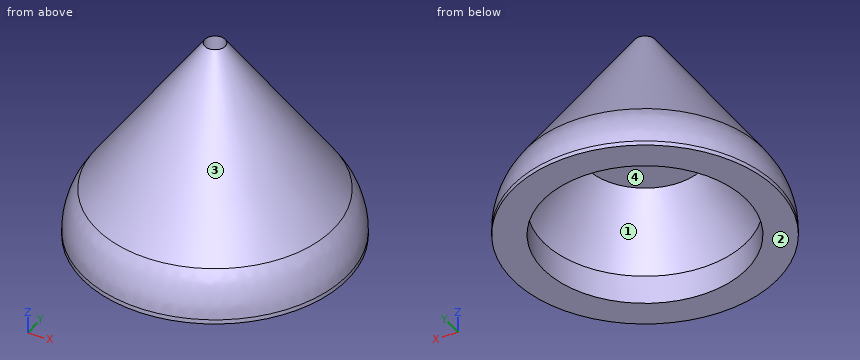
from build123d import *

# Parameters (mm, degrees)
FILLET1_R = 48.26


with BuildPart() as part:
    # Sketch2 → Revolve1 (revolve)
    with BuildSketch(Plane.YZ, mode=Mode.PRIVATE) as revolve1_sk:
        Polygon((-63.5, 0), (-63.5, 17.927965037), (-36.337085401, 56.808731059), (-6.35, 56.808731059), (-6.35, 69.508731059), (-27.464600347, 69.508731059), (-6.35, 99.731991259), (-6.35, 127), (-82.55, 17.927965037), (-82.55, 0), align=None)
    revolve(revolve1_sk.sketch.rotate(Axis((0, 0, 0), (0, 0, 1)), 270), axis=Axis((0, 0, 0), (0, 0, 1)))

    # Fillet1
    fillet1_edges = [part.edges().sort_by_distance(p)[0] for p in [
        (82.55, 0, 17.927965037),
    ]]
    fillet(fillet1_edges, radius=FILLET1_R)


solid = part.part
Work out the finished part from the listing and answer in its coordinate system (mm). Face numbers are marked on the shaded views. Coordinates: 2 decimals unless noted, no trailing zeros. Write each loop counter-clockwise with the first axis right and the second up, starting at its lowest first coordinate (ties: lowest second). Pieces come first, ordered by that corner, then holes. Notation, with made-up numbers: M 17,87.25 L 27,87.25 A22 ccw 27,106.25 Z; hole C 37.5,-4.75 d8. An arc over 180 degrees is marked long. Write item = value, one per line.
1. Straight lines are drawn through the part: line 1 (Y direction, x = 0, z = 4.75); line 2 (X direction, y = 6, z = 39.5); line 3 (Y direction, x = 0, z = 107). For each, find the intervals that lie inside material, in ascending order. Write a range as from..to.
Solution:
line_1 = -82.51..-63.5, 63.5..82.51
line_2 = -67.21..-48.06, 48.06..67.21
line_3 = -20.32..-6.35, 6.35..20.32
2. The part is cut by section A-A (z = 81). Determine the outline of the cut face in (x, y).
Solution:
outline = C 0,0 d76.97; hole C 0,0 d38.87
3. Flat-ended cylindrical pins translate along their axes: pin 1 (1 mm diameter, centred on y = -33, z = 34.5, fed in from +X); pin 2 (5 mm diameter, centred on x = 50.5, y = -63.5, fed in from +Z); pin 3 (10 mm diameter, centred on y = -40, z = 66, fed in from +X). Find the tip coordinate at first contact, or state that the pin passes through.
Solution:
pin_1 = 63.31
pin_2 = 21.79
pin_3 = 36.28
4. Determine the mould class of the marked faces 1, 2, 3 and 4 for opening direction Y: released by +Y, released by -Y, zero draft, split by the parting line, or undercut.
Solution:
face_1 = undercut
face_2 = zero draft
face_3 = split by the parting line
face_4 = undercut
